from build123d import *

# Parameters (mm, degrees)
SKETCH1_W             = 25
SKETCH1_H             = 76.2
EXTRUDE1_DEPTH        = 19.05
M16_CLEARANCE_HOLE1_D = 16.9926
EXTRUDE3_DEPTH        = 50.39142132
M8_CLEARANCE_HOLE1_D  = 9


with BuildPart() as part:
    # Sketch1 → Extrude1 (new, symmetric)
    with BuildSketch(Plane.XY):
        Rectangle(SKETCH1_W, SKETCH1_H)
    extrude(amount=EXTRUDE1_DEPTH, both=True)

    # M16 Clearance Hole1 (through all)
    with Locations(Plane.ZY.offset(12.5)):
        with Locations((0, -20.32), (0, 20.32)):
            Hole(M16_CLEARANCE_HOLE1_D / 2)

    # Sketch2 → Extrude3 (cut, through all)
    with BuildSketch(Plane(origin=(12.5, 0, 0), x_dir=(0, 0, -1), z_dir=(1, 0, 0))):
        Polygon((19.05, 10.5), (7.9629, 10.5), (7.9629, 20), (-7.9629, 20), (-7.9629, -20), (7.9629, -20), (7.9629, -10.5), (19.05, -10.5), align=None)
    extrude(amount=-EXTRUDE3_DEPTH, mode=Mode.SUBTRACT)

    # M8 Clearance Hole1 (through all)
    with Locations(Plane(origin=(12.5, 0, 0), x_dir=(0, 0, -1), z_dir=(1, 0, 0))):
        with Locations((-12, 30), (12, 30), (12, -30), (-12, -30)):
            Hole(M8_CLEARANCE_HOLE1_D / 2)


solid = part.part
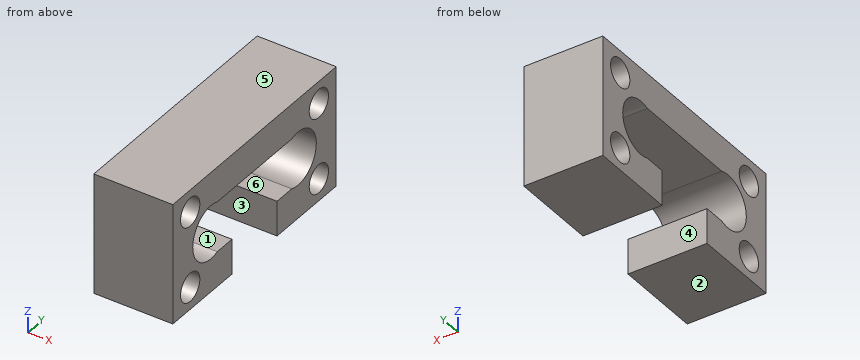
Verification items for the finished model (mm, model axes). Face numbers are marked on the shaded views. A direction names the side the tool comes from. Give positions to 0.01 mm unless a question says otherwise; leave off trailing zeros. Write each loop counter-clockwise with the first axis right and the second up, starting at its lowest first coordinate (ties: lowest second). Pieces come first, ordered by that corner, then holes.
(1) Gauge pin test, flat end, axial feed: pin 1 (10 mm diameter, centred on y = 20.32, z = 0, fed in from -X). Record the tip position at first contact, or that the pin passes through.
(2) Cross-section at C-C (y = 20.32). Enter the section's corners in (x, z), plus the area to 3 significant figures.
(3) Cross-section at A-A (z = -12). Enter the section's corners in (x, y).
(4) Access from +Z, -Z, +X, -X, +Y, -Y to the whole of each face (thin tool, end or side, straight path). Record for the marked faces 4, 5 and 6.
(5) Cross-section at B-B (y = -30). Enter the section's corners in (x, z), plus the area to 4 significant figures.
(6) Cross-section at D-D (z = 12). Enter the section's corners in (x, y), plus the area to 4 significant figures.
(7) Mould release check, pull along Z, two halves, no side actions. Record for the marked faces 1, 2 and 3: +Z half, -Z half, draft (parallel to the pull), parting line (faces both ways), or undercut.
(8) Material ranges on line 1 (Y direction, x = -2.75, z = -12); line 2 (Y direction, x = -6.25, z = 12); line 3 (Y direction, x = -10, z = -10.5), recorded low to high.
Worked out:
1. pin 1: passes through
2. outline: (-12.5, -19.05) - (12.5, -19.05) - (12.5, -8.5) - (-12.5, -8.5) - close; (-12.5, 8.5) - (12.5, 8.5) - (12.5, 19.05) - (-12.5, 19.05) - close
2. area: 528 mm2
3. outline: (-12.5, -38.1) - (12.5, -38.1) - (12.5, -34.5) - (-12.5, -34.5) - close; (-12.5, -25.5) - (12.5, -25.5) - (12.5, -10.5) - (-12.5, -10.5) - close; (-12.5, 10.5) - (12.5, 10.5) - (12.5, 25.5) - (-12.5, 25.5) - close; (-12.5, 34.5) - (12.5, 34.5) - (12.5, 38.1) - (-12.5, 38.1) - close
4. face 4: -Z, +X, -X
4. face 5: +Z, +X, -X, +Y, -Y
4. face 6: +X, -X
5. outline: (-12.5, -19.05) - (12.5, -19.05) - (12.5, -16.5) - (-12.5, -16.5) - close; (-12.5, -7.5) - (12.5, -7.5) - (12.5, 7.5) - (-12.5, 7.5) - close; (-12.5, 16.5) - (12.5, 16.5) - (12.5, 19.05) - (-12.5, 19.05) - close
5. area: 502.5 mm2
6. outline: (-12.5, -38.1) - (12.5, -38.1) - (12.5, -34.5) - (-12.5, -34.5) - close; (-12.5, -25.5) - (12.5, -25.5) - (12.5, 25.5) - (-12.5, 25.5) - close; (-12.5, 34.5) - (12.5, 34.5) - (12.5, 38.1) - (-12.5, 38.1) - close
6. area: 1,455 mm2
7. face 1: undercut
7. face 2: -Z half
7. face 3: draft
8. line 1: y = -38.1 to -34.5, -25.5 to -10.5, 10.5 to 25.5, 34.5 to 38.1
8. line 2: y = -38.1 to -34.5, -25.5 to 25.5, 34.5 to 38.1
8. line 3: y = -38.1 to -34.24, -25.76 to -10.5, 10.5 to 25.76, 34.24 to 38.1
